The figure shows three views and two pictorial views of one solid part (mm, origin at its lowest corner). Answer the questions. A direction names the side the tool comes from. Coordinates: 2 decimals unless noted, no trailing zeros. Loops run counter-clockwise (first coordinate to the right, second up) from the corner with the lowest first, then second, coordinate; pieces in that order, holes last. Notation, with made-up numbers: M -28.5,82 L -13.5,82 A26 ccw -13.5,96 Z; hole C -10,-31.5 d9. An arc over 180 degrees is marked long. Write each question's results on one line, items separated by ' | '.
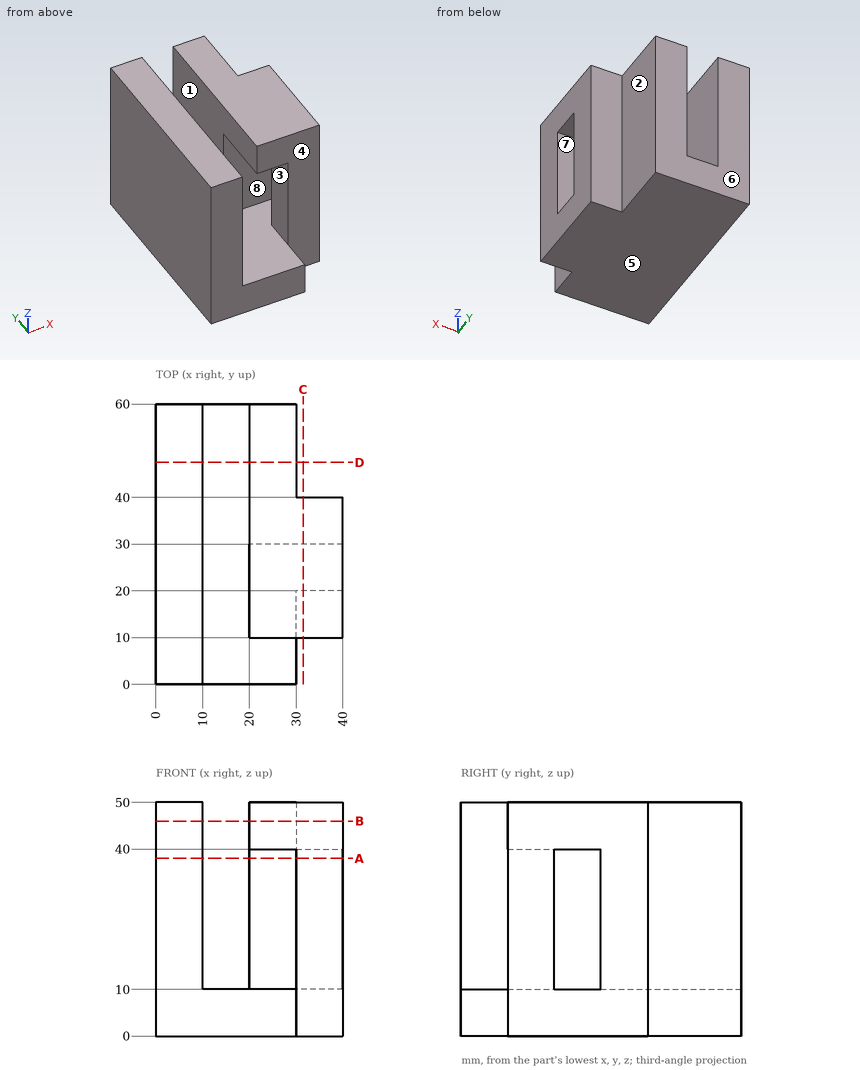
1) Find section C-C, the plane x = 31.5. Give the vertices of the cut face in (y, z).
Check result:
outline: M 10,0 L 40,0 L 40,50 L 10,50 Z; hole M 20,10 L 30,10 L 30,40 L 20,40 Z
2) Given pin 1 Ø16 at (y, z) = (46, 17.5) entering from +X; pin 2 Ø6 at (x, y) = (35, 52) entering from +Z; pin 3 Ø1.5 at (x, z) = (33.5, 34.5) entering from -Y; pin 4 Ø3 at (x, z) = (33, 26) entering from +Y, each flat-ended and moving along its own axis, determine where each tip first touches the part or whether it passes through.
Check result:
pin 1: x = 40 | pin 2: through | pin 3: y = 10 | pin 4: y = 40
3) Find section B-B, the plane z = 46. Give the vertices of the cut face in (x, y), and give its area (3 significant figures).
Check result:
outline: M 0,0 L 10,0 L 10,60 L 0,60 Z; M 20,10 L 40,10 L 40,40 L 30,40 L 30,60 L 20,60 Z | area: 1,400 mm^2
4) Which of the six approach directions +Z, -Z, +X, -X, +Y, -Y give full straight-line access (tool end or side, diameter ignored) to the marked faces 1, 2, 3 and 4?
Check result:
face 1: +Z, +Y, -Y | face 2: +Z, -Z, +X, +Y | face 3: -Y | face 4: +Z, +X, -Y
5) For a pull along Y with two mould halves and no side action, classify the marked faces 5, 6, 7 and 8 as released by +Y, released by -Y, zero draft, split by the parting line, or undercut.
Check result:
face 5: zero draft | face 6: released by +Y | face 7: undercut | face 8: undercut
6) Find section D-D, the plane y = 47.5. Give the vertices of the cut face in (x, z).
Check result:
outline: M 0,0 L 30,0 L 30,50 L 20,50 L 20,10 L 10,10 L 10,50 L 0,50 Z
7) Find section A-A, the plane z = 38. Give the vertices of the cut face in (x, y).
Check result:
outline: M 0,0 L 10,0 L 10,60 L 0,60 Z; M 20,30 L 40,30 L 40,40 L 30,40 L 30,60 L 20,60 Z; M 30,10 L 40,10 L 40,20 L 30,20 Z
8) Straight lines are drawn through the part: probe 1 along Y at (x, z) = (32, 38.5); probe 2 along X at (y, z) = (45, 24); probe 3 along X at (y, z) = (25, 38.5). For each, find the intervals that lie inside material, in ascending order. Write a range as [from, to].
Check result:
probe 1: [10, 20], [30, 40] | probe 2: [0, 10], [20, 30] | probe 3: [0, 10]
